from build123d import *

# Parameters (mm, degrees)
CROQUIS2_W              = 60
CROQUIS2_H              = 60
SALIENTE_EXTRUIR1_DEPTH = 60
CORTAR_EXTRUIR1_DEPTH   = 40


with BuildPart() as part:
    # Croquis2 → Saliente-Extruir1 (new body)
    with BuildSketch(Plane(origin=(0, 0, 0), x_dir=(1, 0, 0), z_dir=(0, 1, 0))):
        with Locations((30, 30)):
            Rectangle(CROQUIS2_W, CROQUIS2_H)
    extrude(amount=SALIENTE_EXTRUIR1_DEPTH)

    # Croquis3 → Cortar-Extruir1 (cut)
    with BuildSketch(Plane.XY):
        Polygon((60, 0), (20, 30), (20, 60), (60, 60), align=None)
    extrude(amount=-CORTAR_EXTRUIR1_DEPTH, mode=Mode.SUBTRACT)


solid = part.part
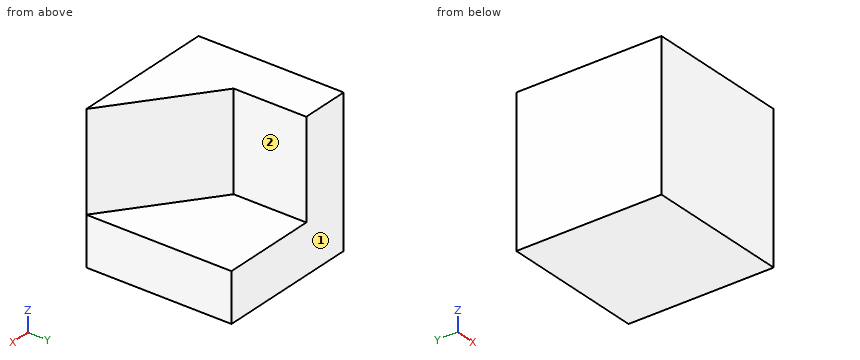
Verification items for the finished model (mm, model axes). Face numbers are marked on the shaded views. A direction names the side the tool comes from. Coordinates: 2 decimals unless noted, no trailing zeros. Order: outer loops, then holes, each group sorted by start corner. A loop starts at its lowest first (then second) coordinate and runs counter-clockwise, first axis right, second up.
1. Sectioned sample at A-A, the plane y = 42. Record the cut outline in (x, z), and give its area (3 significant figures).
Results found:
outline: (0, -60) - (60, -60) - (60, -40) - (20, -40) - (20, 0) - (0, 0) - close
area: 2,000 mm2
2. Sectioned sample at B-B, the plane z = -19. Record the cut outline in (x, y), and give its area (3 significant figures).
Results found:
outline: (0, 0) - (60, 0) - (20, 30) - (20, 60) - (0, 60) - close
area: 1,800 mm2
3. Scan lines: line 1 (Z direction, x = 44, y = 39.5); line 2 (X direction, y = 36.5, z = -4); line 3 (Y direction, x = 41, z = -13.5). Record each from-to range of solid material in increasing order.
Results found:
line 1: z = -60 to -40
line 2: x = 0 to 20
line 3: y = 0 to 14.25
4. Go/stop test with flat-tipped pins: pin 1 Ø10 at (x, y) = (40, 50) entering from +Z; pin 2 Ø9 at (y, z) = (51, -26) entering from +X; pin 3 Ø8 at (x, z) = (43, -8) entering from +Y. Record where each tip stops, or that it passes through.
Results found:
pin 1: stops at z = -40
pin 2: stops at x = 20
pin 3: stops at y = 15.75
5. Set-up check for the marked faces 1 and 2: record each of +Z, -Z, +X, -X, +Y, -Y from which the full face is reachable in a straight line by a thin tool's end or side.
Results found:
face 1: +Z, -Z, +X, -X, +Y
face 2: +Z, +X, +Y
6. Sectioned sample at C-C, the plane x = 43. Record the cut outline in (y, z).
Results found:
outline: (0, -60) - (60, -60) - (60, -40) - (12.75, -40) - (12.75, 0) - (0, 0) - close
